Work out the finished part from the listing and answer in its coordinate system (mm). Face numbers are marked on the shaded views. A direction names the side the tool comes from. Coordinates: 2 decimals unless noted, no trailing zeros. Loops run counter-clockwise (first coordinate to the right, second up) from the corner with the lowest first, then second, coordinate; pieces in that order, holes last. Notation, with made-up numbers: M 21,-9 L 44,-9 A14 cw 44,14 Z; hole C -1.75,-40 d7. An arc over 180 degrees is marked long. Write each question's results on one line, items separated by ' | '.
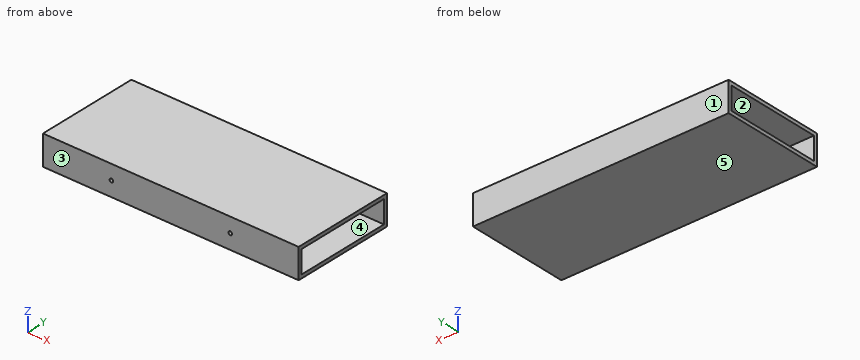
```python
from build123d import *

# Parameters (mm, degrees)
SKETCH1_W           = 215
SKETCH1_H           = 25
BOSS_EXTRUDE1_DEPTH = 87
SKETCH3_W           = 19
SKETCH3_H           = 81
CUT_EXTRUDE1_DEPTH  = 216
SKETCH4_R           = 1.5
CUT_EXTRUDE2_DEPTH  = 3


with BuildPart() as part:
    # Sketch1 → Boss-Extrude1 (new body)
    with BuildSketch(Plane(origin=(0, 0, 0), x_dir=(1, 0, 0), z_dir=(0, 1, 0))):
        Rectangle(SKETCH1_W, SKETCH1_H)
    extrude(amount=BOSS_EXTRUDE1_DEPTH)

    # Sketch3 → Cut-Extrude1 (cut, through all)
    with BuildSketch(Plane.ZY.offset(107.5)):
        with Locations((0, 43.5)):
            Rectangle(SKETCH3_W, SKETCH3_H)
    extrude(amount=-CUT_EXTRUDE1_DEPTH, mode=Mode.SUBTRACT)

    # Sketch4 → Cut-Extrude2 (cut)
    with BuildSketch(Plane.XZ):
        with Locations((-50, 0)):
            Circle(SKETCH4_R)
        with Locations((50, 0)):
            Circle(SKETCH4_R)
    extrude(amount=-CUT_EXTRUDE2_DEPTH, mode=Mode.SUBTRACT)


solid = part.part
```
1) Straight lines are drawn through the part: probe 1 along Z at (x, y) = (87.5, 40); probe 2 along Y at (x, z) = (-27.5, -0.25); probe 3 along Z at (x, y) = (50, 2.15). For each, find the intervals that lie inside material, in ascending order. Write a range as [from, to].
Check result:
probe 1: [-12.5, -9.5], [9.5, 12.5] | probe 2: [0, 3], [84, 87] | probe 3: [-12.5, -1.5], [1.5, 12.5]
2) Find section A-A, the plane z = -7. Give the vertices of the cut face in (x, y).
Check result:
outline: M -107.5,0 L 107.5,0 L 107.5,3 L -107.5,3 Z; M -107.5,84 L 107.5,84 L 107.5,87 L -107.5,87 Z
3) Given pin 1 Ø2.5 at (x, z) = (50, 0) entering from -Y, flat-ended and moving along its own axis, determine where the tip first touches the part or whether it passes through.
Check result:
pin 1: y = 84
4) Find section C-C, the plane x = 11.5. Give the vertices of the cut face in (y, z), and give its area (3 significant figures).
Check result:
outline: M 0,-12.5 L 87,-12.5 L 87,12.5 L 0,12.5 Z; hole M 3,-9.5 L 84,-9.5 L 84,9.5 L 3,9.5 Z | area: 636 mm^2
5) For a pull along Y with two mould halves and no side action, classify the marked faces 3, 4 and 5 as released by +Y, released by -Y, zero draft, split by the parting line, or undercut.
Check result:
face 3: released by -Y | face 4: undercut | face 5: zero draft
6) Find section B-B, the plane y = 29.5. Give the vertices of the cut face in (x, z).
Check result:
outline: M -107.5,-12.5 L 107.5,-12.5 L 107.5,-9.5 L -107.5,-9.5 Z; M -107.5,9.5 L 107.5,9.5 L 107.5,12.5 L -107.5,12.5 Z
7) Which of the six approach directions +Z, -Z, +X, -X, +Y, -Y give full straight-line access (tool end or side, diameter ignored) to the marked faces 1 and 2?
Check result:
face 1: +Z, -Z, +X, -X, +Y | face 2: +X, -X
